The listing builds one solid part. Answer for the finished solid, in the listing's coordinates (mm). Round coordinates to 2 decimals unless told otherwise and drop trailing zeros. Write each loop counter-clockwise with the first axis right and the second up, starting at its lowest first coordinate (ties: lowest second). Pieces come first, ordered by that corner, then holes.
Item 1: Find section B-B on z = -16.5. Give the vertices of the cut face in (x, y), then the cut area to 3 significant figures.
Item 2: Find section C-C on x = 35. Give the vertices of the cut face in (y, z).
Item 3: Find the intervals of material crossed by probe 1 along X at (y, z) = (1.45, 12); probe 2 along X at (y, z) = (1.45, 0); probe 3 along Z at (x, y) = (-7, 0.15), in increasing order.
Item 4: Find section A-A on z = 12. Give the vertices of the cut face in (x, y), then the cut area to 3 significant figures.
Item 5: Find section D-D on y = 1.35. Give the number of separate pieces and of enclosed holes in the cut face, then the cut area to 3 significant figures.
```python
from build123d import *

# Parameters (mm, degrees)
SKETCH_1_W      = 100
SKETCH_1_H      = 140
SKETCH_1_R      = 1.6
SKETCH_1_W_2    = 56
SKETCH_1_H_2    = 120
EXTRUDE_1_DEPTH = 2
FILLET_1_R      = 28


with BuildPart() as part:
    # 草圖1 → 填料-伸長1 (new body)
    with BuildSketch(Plane(origin=(0, 0, 0), x_dir=(1, 0, 0), z_dir=(0, 1, 0))):
        Rectangle(SKETCH_1_W, SKETCH_1_H)
        with Locations(Location((-35, 30, 0), (0, 0, 270))):
            Circle(SKETCH_1_R, mode=Mode.SUBTRACT)
        with Locations(Location((35, 30, 0), (0, 0, 90))):
            Circle(SKETCH_1_R, mode=Mode.SUBTRACT)
        with Locations(Location((-35, 12, 0), (0, 0, 270))):
            Circle(SKETCH_1_R, mode=Mode.SUBTRACT)
        with Locations(Location((35, 12, 0), (0, 0, 90))):
            Circle(SKETCH_1_R, mode=Mode.SUBTRACT)
        with Locations(Location((35, -12, 0), (0, 0, 270))):
            Circle(SKETCH_1_R, mode=Mode.SUBTRACT)
        with Locations(Location((35, -30, 0), (0, 0, 270))):
            Circle(SKETCH_1_R, mode=Mode.SUBTRACT)
        with Locations(Location((-35, -30, 0), (0, 0, 90))):
            Circle(SKETCH_1_R, mode=Mode.SUBTRACT)
        with Locations(Location((-35, -12, 0), (0, 0, 90))):
            Circle(SKETCH_1_R, mode=Mode.SUBTRACT)
        Rectangle(SKETCH_1_W_2, SKETCH_1_H_2, mode=Mode.SUBTRACT)
    extrude(amount=EXTRUDE_1_DEPTH)

    # 圓角1
    fillet_1_edges = [part.edges().sort_by_distance(p)[0] for p in [
        (28, 1, -60),
        (-28, 1, -60),
        (-28, 1, 60),
        (28, 1, 60),
    ]]
    fillet(fillet_1_edges, radius=FILLET_1_R - 0.0001)  # a hair under: the kernel refuses the full size


solid = part.part
```
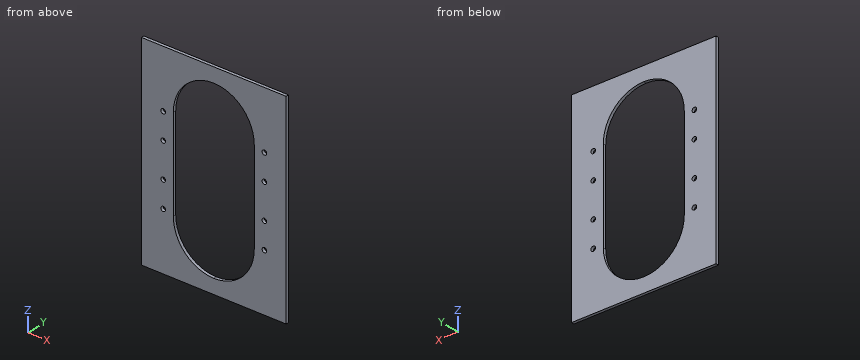
Check values:
1. outline: (-50, 0) - (-28, 0) - (-28, 2) - (-50, 2) - close; (28, 0) - (50, 0) - (50, 2) - (28, 2) - close
1. area: 88.0 mm2
2. outline: (0, -70) - (2, -70) - (2, -31.6) - (0, -31.6) - close; (0, -28.4) - (2, -28.4) - (2, -13.6) - (0, -13.6) - close; (0, -10.4) - (2, -10.4) - (2, 10.4) - (0, 10.4) - close; (0, 13.6) - (2, 13.6) - (2, 28.4) - (0, 28.4) - close; (0, 31.6) - (2, 31.6) - (2, 70) - (0, 70) - close
3. probe 1: x = -50 to -36.6, -33.4 to -28, 28 to 33.4, 36.6 to 50
3. probe 2: x = -50 to -28, 28 to 50
3. probe 3: z = -70 to -59.11, 59.11 to 70
4. outline: (-50, 0) - (-36.6, 0) - (-36.6, 2) - (-50, 2) - close; (-33.4, 0) - (-28, 0) - (-28, 2) - (-33.4, 2) - close; (28, 0) - (33.4, 0) - (33.4, 2) - (28, 2) - close; (36.6, 0) - (50, 0) - (50, 2) - (36.6, 2) - close
4. area: 75.2 mm2
5. separate pieces: 1
5. enclosed holes: 9
5. area: 7,890 mm2
